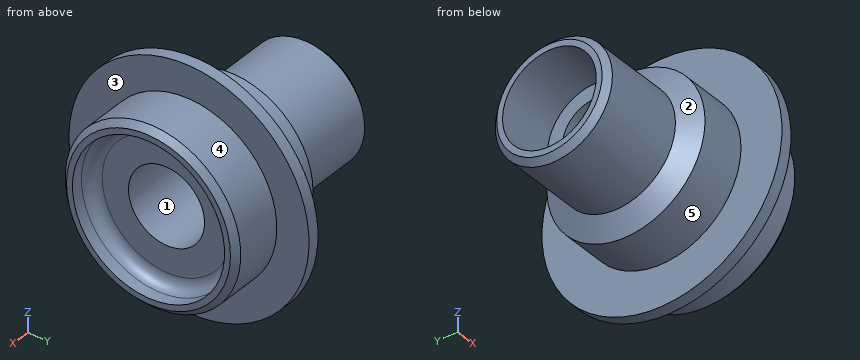
```python
from build123d import *

# Parameters (mm, degrees)
CHAMFER1_SIZE = 1


with BuildPart() as part:
    # Sketch2 → Revolve1 (revolve)
    with BuildSketch(Plane.XY, mode=Mode.PRIVATE) as revolve1_sk:
        with BuildLine():
            Line((0, 8), (0, 10))
            Line((0, 10), (15, 10))
            Line((15, 10), (17.020725942, 13.5))
            Line((17.020725942, 13.5), (25, 13.5))
            Line((25, 13.5), (25, 20.5))
            Line((25, 20.5), (27, 20.5))
            Line((27, 20.5), (27, 15))
            Line((27, 15), (36, 15))
            Line((36, 15), (36, 13))
            Line((36, 13), (34, 13))
            ThreePointArc((34, 13), (32.585786438, 12.414213562), (32, 11))
            Line((32, 11), (32, 6.5))
            Line((32, 6.5), (12, 6.5))
            Line((12, 6.5), (12, 5.5))
            Line((12, 5.5), (10, 5.5))
            Line((10, 5.5), (10, 8))
            Line((10, 8), (0, 8))
        make_face()
    revolve(revolve1_sk.sketch.rotate(Axis((0, 0, 0), (1, 0, 0)), 90), axis=Axis((0, 0, 0), (1, 0, 0)))

    # Chamfer1
    chamfer1_edges = [part.edges().sort_by_distance(p)[0] for p in [
        (0, 0, -10),
        (36, 0, -15),
    ]]
    chamfer(chamfer1_edges, length=CHAMFER1_SIZE)


solid = part.part
```
Design review of the part built by this model. Coordinates are the model's own, in mm. Face numbers are marked on the shaded views. A direction names the side the tool comes from. Round coordinates to 2 decimals unless told otherwise and drop trailing zeros. Write each loop counter-clockwise with the first axis right and the second up, starting at its lowest first coordinate (ties: lowest second). Pieces come first, ordered by that corner, then holes.
Item 1: The part is to be moulded in two halves that separate along Y. For the marked faces 1, 2 and 3, say which applies: +Y half, -Y half, draft (parallel to the pull), parting line (faces both ways), or undercut.
Item 2: We need section C-C on y = -17. Write out the cut boundary in (x, z), and give its area (3 significant figures).
Item 3: Clearance check with flat-ended pins moving along their axes: pin 1 Ø11 at (y, z) = (-3.5, 0.5) entering from +X; pin 2 Ø3 at (x, z) = (13.5, 2.5) entering from -Y; pin 3 Ø1.5 at (x, y) = (14.5, 14) entering from +Z; pin 4 Ø6 at (x, y) = (20, 14) entering from -Z. State where each tip first meets the part, or that it passes through.
Item 4: We need section B-B on x = 23.5. Write out the cut boundary in (y, z).
Item 5: We need section A-A on x = 3.5. Write out the cut boundary in (y, z), and give its area (3 significant figures).
Item 6: For the marked faces 4 and 5, list the 3-axis set-ups (+Z, -Z, +X, -X, +Y, -Y) from which the entire face can be reached by the end or side of a thin tool; tool diameter is ignored.
Item 7: For probe 1 along Y at (x, z) = (24.75, 0); probe 2 along X at (y, z) = (-14, -13); probe 3 along X at (y, z) = (12, 7), list the stretches that pass through material, from the lowest coordinate up.
Returned:
1. face 1: undercut
1. face 2: parting line
1. face 3: draft
2. outline: (25, -11.46) - (27, -11.46) - (27, 11.46) - (25, 11.46) - close
2. area: 45.8 mm2
3. pin 1: stops at x = 32
3. pin 2: stops at y = -9.95
3. pin 3: passes through
3. pin 4: stops at z = -7.83
4. outline: circle Ø27 at (0, 0); hole circle Ø13 at (0, 0)
5. outline: circle Ø20 at (0, 0); hole circle Ø16 at (0, 0)
5. area: 113 mm2
6. face 4: +X
6. face 5: -X
7. probe 1: y = -13.5 to -6.5, 6.5 to 13.5
7. probe 2: x = 25 to 27
7. probe 3: x = 25 to 36
